Could you check a few things on this model? Use its own coordinates, in mm. A direction names the side the tool comes from. Round coordinates to 2 decimals unless told otherwise and drop trailing zeros. Loops run counter-clockwise (first coordinate to the right, second up) from the corner with the lowest first, then second, coordinate; pieces in that order, holes last. Notation, with made-up numbers: M 4,27.25 L 29,27.25 A20 ccw 29,48.25 Z; hole C -35.75,49 d5. An arc over 180 degrees is marked long. One line per item, written item: value. Start each with the question number.
Q1. Thinking about a two-plate mould opening in Y: for faces 6 (the face through (-2, 6.6, -6)), 7 (the face through (0, 11, -4)), 8 (the face through (1, 11, 0)), which applies, released by +Y, released by -Y, zero draft, split by the parting line, or undercut?
Q2. Please list where these lines run through material, in increasing order: line 1 along Y through (x, z) = (-5.7, -10.6); line 2 along Y through (x, z) = (0, -2.75); line 3 along Z through (x, y) = (-5.5, 12).
Q3. Imagine slicing it at D-D (z = -3.75). Please give me the cut outline in (x, y).
Q4. Imagine slicing it at B-B (x = 0). Please give me the cut outline in (y, z).
Q5. I'm going to push flat-ended pins straight in: pin 1 Ø4 at (y, z) = (13.5, -12.5) entering from +X; pin 2 Ø2.5 at (y, z) = (13.5, -5.5) entering from +X; pin 3 Ø5 at (x, y) = (0.5, 9) entering from +Z; pin 4 Ø4 at (x, y) = (3.5, 13.5) entering from -Z. Where does each tip first touch, or does it pass through?
Q6. Which directions (+Z, -Z, +X, -X, +Y, -Y) give clear straight access to the entire face, cutting with the end or side of a thin tool? Please do faces 1 (the face through (-2, 8, -10)), 2 (the face through (-4, 12, -3)), 3 (the face through (-4, 16.657, -13)), 4 (the face through (4, 12, -4.6)), 5 (the face through (-4, 12, -7)).
Q7. Imagine slicing it at A-A (x = -5.5). Please give me the cut outline in (y, z), then the cut area to 3 significant figures.
Q8. Imagine slicing it at C-C (y = 12.5). Please give me the cut outline in (x, z).
from build123d import *

# Parameters (mm, degrees)
BOSS_EXTRUDE1_DEPTH      = 25
CUT_EXTRUDE1_REACH       = 27
M3_TAPPED_HOLE1_D        = 3
M3_TAPPED_HOLE1_DEPTH    = 7.5
M4_CLEARANCE_HOLE1_D     = 4.5
M4_CLEARANCE_HOLE1_DEPTH = 4.5
CUT_EXTRUDE2_DEPTH       = 3.3
SKETCH9_W                = 12.3
SKETCH9_H                = 6.6
CUT_EXTRUDE3_DEPTH       = 15.6


with BuildPart() as part:
    # Sketch1 → Boss-Extrude1 (new body)
    with BuildSketch(Plane(origin=(0, 0, 0), x_dir=(1, 0, 0), z_dir=(0, 1, 0))):
        Polygon((-3.8, 0), (-5.8, 2), (-5.8, 3), (-2, 3), (-2, 4.6), (-6.5, 4.6), (-6.5, 14.6), (6.5, 14.6), (6.5, 4.6), (2, 4.6), (2, 3), (5.8, 3), (5.8, 2), (3.8, 0), align=None)
    extrude(amount=BOSS_EXTRUDE1_DEPTH)

    # Sketch2 → Cut-Extrude1 (cut, up to next)
    with BuildSketch(Plane(origin=(0, 25, 0), x_dir=(1, 0, 0), z_dir=(0, 1, 0)), mode=Mode.PRIVATE) as cut_extrude1_sk1:
        Polygon((6.5, 4.6), (5, 4.6), (5, 7.5), (-2, 7.5), (-2, 14.6), (6.5, 14.6), align=None)
    cut_extrude1_tool1 = extrude(cut_extrude1_sk1.sketch, amount=-CUT_EXTRUDE1_REACH, mode=Mode.PRIVATE) & part.part
    add(cut_extrude1_tool1.solids().sort_by_distance((2.485317, 25, -10.713833))[0], mode=Mode.SUBTRACT)

    # M3 Tapped Hole1
    with Locations(Plane(origin=(0, 0, -7.5), x_dir=(-1, 0, 0), z_dir=(0, 0, -1))):
        with Locations((0, 22), (0, 3), (0, 12.5)):
            Hole(M3_TAPPED_HOLE1_D / 2, depth=M3_TAPPED_HOLE1_DEPTH)

    # M4 Clearance Hole1
    with Locations(Plane.ZY.offset(6.5)):
        with Locations((-10.6, 12.5)):
            Hole(M4_CLEARANCE_HOLE1_D / 2, depth=M4_CLEARANCE_HOLE1_DEPTH)

    # Sketch8 → Cut-Extrude2 (cut)
    with BuildSketch(Plane(origin=(-2, 0, 0), x_dir=(0, 0, -1), z_dir=(1, 0, 0))):
        Polygon((10.6, 16.656921938), (14.6, 16.656921938), (14.6, 8.343078062), (10.6, 8.343078062), (7, 10.421539031), (7, 14.578460969), align=None)
    extrude(amount=-CUT_EXTRUDE2_DEPTH, mode=Mode.SUBTRACT)

    # Sketch9 → Cut-Extrude3 (cut, through all)
    with BuildSketch(Plane(origin=(0, 0, -14.6), x_dir=(-1, 0, 0), z_dir=(0, 0, -1))):
        with Locations((0.35, 21.7)):
            Rectangle(SKETCH9_W, SKETCH9_H)
        with Locations((0.35, 3.3)):
            Rectangle(SKETCH9_W, SKETCH9_H)
    extrude(amount=-CUT_EXTRUDE3_DEPTH, mode=Mode.SUBTRACT)


solid = part.part
Report:
1. face 6: released by -Y
1. face 7: undercut
1. face 8: zero draft
2. line 1: y = 6.6 to 10.25, 14.75 to 18.4
2. line 2: y = 6.6 to 11, 14 to 18.4
2. line 3: z = -14.6 to -12.79, -8.41 to -4.6, -3 to -1.7
3. outline: M -2,6.6 L 2,6.6 L 2,18.4 L -2,18.4 Z; hole C 0,12.5 d3
4. outline: M 6.6,-7.5 L 11,-7.5 L 11,0 L 6.6,0 Z; M 14,-7.5 L 18.4,-7.5 L 18.4,0 L 14,0 Z
5. pin 1: stops at x = -5.3
5. pin 2: stops at x = 5
5. pin 3: stops at z = 0
5. pin 4: stops at z = -7.5
6. face 1: -Z, +X, +Y, -Y
6. face 2: -X, +Y, -Y
6. face 3: -Z, +X
6. face 4: +X, +Y, -Y
6. face 5: -Z
7. outline: M 6.6,-14.6 L 18.4,-14.6 L 18.4,-4.6 L 6.6,-4.6 Z; M 6.6,-3 L 18.4,-3 L 18.4,-1.7 L 6.6,-1.7 Z; hole C 12.5,-10.6 d4.5
7. area: 117 mm²
8. outline: M -6.5,-14.6 L -5.3,-14.6 L -5.3,-12.85 L -6.5,-12.85 Z; M -6.5,-8.35 L -5.3,-8.35 L -5.3,-7 L -2,-7 L -2,-7.5 L -1.5,-7.5 L -1.5,0 L -3.8,0 L -5.8,-2 L -5.8,-3 L -2,-3 L -2,-4.6 L -6.5,-4.6 Z; M 1.5,-7.5 L 5,-7.5 L 5,-4.6 L 2,-4.6 L 2,-3 L 5.8,-3 L 5.8,-2 L 3.8,0 L 1.5,0 Z
